Autodesk Inventor part; units mm, degrees
ref_plane "YZ Plane" through (0, 0, 0) normal (1, 0, 0) x (0, 1, 0)
ref_plane "XZ Plane" through (0, 0, 0) normal (0, 1, 0) x (-1, 0, 0)
ref_plane "XY Plane" through (0, 0, 0) normal (0, 0, 1) x (1, 0, 0)
sketch "Sketch1" plane through (0, 0, 0) normal (0, 1, 0) x (-1, 0, 0)
  line L0 (45, 12.5) -> (-45, 12.5)
  line L1 (-45, 12.5) -> (-45, -12.5)
  line L2 (-45, -12.5) -> (45, -12.5)
  line L3 (45, -12.5) -> (45, 12.5)
  line L4 (45, 12.5) -> (-45, -12.5) construction
  line L5 (-45, 12.5) -> (45, -12.5) construction
  line L6 (43, 10.5) -> (-43, 10.5)
  line L7 (-43, 10.5) -> (-43, -10.5)
  line L8 (-43, -10.5) -> (43, -10.5)
  line L9 (43, -10.5) -> (43, 10.5)
  line L10 (43, 10.5) -> (-43, -10.5) construction
  line L11 (-43, 10.5) -> (43, -10.5) construction
  point P0 (0, 0)
  dimension "d0" = 90
  dimension "d1" = 25
  dimension "d2" = 86
  dimension "d3" = 21
extrude "Extrusion1" add sketch "Sketch1" along normal blind 50
sketch "Sketch2" plane through (-45, 0, 12.5) normal (0, 0, 1) x (1, 0, 0)
  circle A0 centre (45, 25) radius 9.8
  line L0 (90, 0) -> (90, 50)
  line L1 (0, 50) -> (90, 50)
  point P0 (45, 0)
  dimension "d6" = 19.6
  dimension "d7" = 45
  dimension "d8" = 25
extrude "Extrusion2" cut sketch "Sketch2" against normal blind 29.05
sketch "Sketch3" plane through (45, 0, 12.5) normal (1, 0, 0) x (0, 0, -1)
  circle A0 centre (19.5, 10) radius 2.65
  circle A1 centre (5.5, 10) radius 2.65
  circle A2 centre (19.5, 40) radius 2.65
  circle A3 centre (5.5, 40) radius 2.65
  line L0 (0, 50) -> (25, 50)
  line L1 (25, 0) -> (25, 50)
  line L2 (0, 0) -> (0, 50)
  line L3 (0, 0) -> (25, 0)
  point P0 (12.5, 0)
  dimension "d11" = 5.3
  dimension "d12" = 5.3
  dimension "d13" = 5.3
  dimension "d14" = 5.3
  dimension "d15" = 10
  dimension "d16" = 10
  dimension "d17" = 5.5
  dimension "d18" = 5.5
  dimension "d19" = 10
  dimension "d20" = 5.5
  dimension "d21" = 5.5
  dimension "d22" = 10
extrude "Extrusion3" cut sketch "Sketch3" against normal blind 143.35 contours A0 | A1 | A2 | A3
properties part number "Bevel holder"
The listing builds one solid part. Answer for the finished solid, in the listing's coordinates (mm). A direction names the side the tool comes from. Round coordinates to 2 decimals unless told otherwise and drop trailing zeros. Order: outer loops, then holes, each group sorted by start corner. A loop starts at its lowest first (then second) coordinate and runs counter-clockwise, first axis right, second up. Notation, with made-up numbers: (80.25, 83) -> (120.25, 83) arc R17 ccw to (120.25, 101) -> close; hole circle Ø11 at (30, -7). An arc over 180 degrees is marked (long way). One line per item, written item: value.
Item 1: For a pull along X with two mould halves and no side action, classify faces 1 (the cylindrical face through (-43.986, 10.117, 9.647)), 2 (the flat face through (-43, 25, 0)), 3 (the flat face through (-10, 25, 10.5)), 4 (the flat face through (-45, 25, 0)) as released by +X, released by -X, zero draft, split by the parting line, or undercut.
Taken from the geometry:
face 1: zero draft
face 2: undercut
face 3: undercut
face 4: released by -X
Item 2: Straight lines are drawn through the part: L1, parallel to Y at x = 43.5, z = 7; L2, parallel to Z at x = -29.5, y = 27; L3, parallel to X at y = 37, z = 8.5. For each, find the intervals that lie inside material, in ascending order.
Taken from the geometry:
L1: y = 0 to 7.35, 12.65 to 37.35, 42.65 to 50
L2: z = -12.5 to -10.5, 10.5 to 12.5
L3: x = -45 to -43, 43 to 45
Item 3: Given P1, Ø6, axis at y = 10, z = 7, coming from the -X side; P2, Ø5, axis at y = 10, z = 7, coming from the +X side, each flat-ended and moving along its own axis, determine where each tip first touches the part or whether it passes through.
Taken from the geometry:
P1: stops at x = -45
P2: passes through
Item 4: Find section C-C, the plane x = 29. Give the vertices of the cut face in (y, z), then the cut area to 3 significant figures.
Taken from the geometry:
outline: (0, -12.5) -> (50, -12.5) -> (50, -10.5) -> (0, -10.5) -> close; (0, 10.5) -> (50, 10.5) -> (50, 12.5) -> (0, 12.5) -> close
area: 200 mm2
Item 5: Find section D-D, the plane z = 7. Give the vertices of the cut face in (x, y).
Taken from the geometry:
outline: (-45, 0) -> (-43, 0) -> (-43, 7.35) -> (-45, 7.35) -> close; (-45, 12.65) -> (-43, 12.65) -> (-43, 37.35) -> (-45, 37.35) -> close; (-45, 42.65) -> (-43, 42.65) -> (-43, 50) -> (-45, 50) -> close; (43, 0) -> (45, 0) -> (45, 7.35) -> (43, 7.35) -> close; (43, 12.65) -> (45, 12.65) -> (45, 37.35) -> (43, 37.35) -> close; (43, 42.65) -> (45, 42.65) -> (45, 50) -> (43, 50) -> close
Item 6: Find section B-B, the plane y = 6.5. Give the vertices of the cut face in (x, z), then the cut area to 3 significant figures.
Taken from the geometry:
outline: (-45, -12.5) -> (45, -12.5) -> (45, 12.5) -> (-45, 12.5) -> close; hole (-43, -10.5) -> (43, -10.5) -> (43, 10.5) -> (-43, 10.5) -> close
area: 444 mm2
Item 7: For faces 5 (the cylindrical face through (-43.99, 42.63, -6.66)), 6 (the flat face through (10, 25, -10.5)), determine the directions among +Z, -Z, +X, -X, +Y, -Y from which every point of the face is accessible in a straight line to the end or side of a thin tool.
Taken from the geometry:
face 5: +X, -X
face 6: +Y, -Y
Item 8: Find section A-A, the plane z = -3. Give the vertices of the cut face in (x, y), then the cut area to 3 significant figures.
Taken from the geometry:
outline: (-45, 0) -> (-43, 0) -> (-43, 50) -> (-45, 50) -> close; (43, 0) -> (45, 0) -> (45, 50) -> (43, 50) -> close
area: 200 mm2
